```python
from build123d import *

# Parameters (mm, degrees)
SKETCH_1_R          = 5
EXTRUDE_1_DEPTH     = 5
CUT_EXTRUDE_1_DEPTH = 102.523396318


with BuildPart() as part:
    # 草图1 → 凸台-拉伸1 (new body)
    with BuildSketch(Plane.XY):
        with BuildLine():
            Line((0, 9), (92, 9))
            ThreePointArc((92, 9), (101, 0), (92, -9))
            Line((92, -9), (0, -9))
            ThreePointArc((0, -9), (-9, 0), (0, 9))
        make_face()
        Circle(SKETCH_1_R, mode=Mode.SUBTRACT)
        with Locations((92, 0)):
            Circle(SKETCH_1_R, mode=Mode.SUBTRACT)
    extrude(amount=EXTRUDE_1_DEPTH)

    # 草图2 → 切除-拉伸1 (cut, through all)
    with BuildSketch(Plane.XY.offset(5)):
        with BuildLine():
            Line((9.539392014, 4), (82.460607986, 4))
            ThreePointArc((82.460607986, 4), (83.266833761, 3.591607978), (83.414547187, 2.7))
            ThreePointArc((83.414547187, 2.7), (83, 0), (83.414547187, -2.7))
            ThreePointArc((83.414547187, -2.7), (83.266833761, -3.591607978), (82.460607986, -4))
            Line((82.460607986, -4), (9.539392014, -4))
            ThreePointArc((9.539392014, -4), (8.733166239, -3.591607978), (8.585452813, -2.7))
            ThreePointArc((8.585452813, -2.7), (9, 0), (8.585452813, 2.7))
            ThreePointArc((8.585452813, 2.7), (8.733166239, 3.591607978), (9.539392014, 4))
        make_face()
    extrude(amount=-CUT_EXTRUDE_1_DEPTH, mode=Mode.SUBTRACT)


solid = part.part
```
Work out the finished part from the listing and answer in its coordinate system (mm). A direction names the side the tool comes from. Give positions to 0.01 mm unless a question says otherwise; leave off trailing zeros. Loops run counter-clockwise (first coordinate to the right, second up) from the corner with the lowest first, then second, coordinate; pieces in that order, holes last. Notation, with made-up numbers: (-30, 10) - (22, 10) arc R31 ccw to (22, 46) - close; hole circle Ø6 at (49, -35.75). An arc over 180 degrees is marked (long way). Use CSV: the item, a comma, the result in double quotes. Start each with the question number.
(1) Find section A-A, the plane x = 73.5. Determine the outline of the cut face in (y, z).
(2) A tool of negligible diameter and unlimited length cuts with its end or side. For faces 1 (the face through (45, 4, 3)), 2 (the face through (47, 6, 5)), from which of +Z, -Z, +X, -X, +Y, -Y can it reach the whole face along a straight path? Write none if from no direction.
(3) Find section B-B, the plane y = 0. Determine the outline of the cut face in (x, z), plus the area to 3 significant figures.
(4) Find section C-C, the plane z = 3.4. Determine the outline of the cut face in (x, y), plus the area to 3 significant figures.
(5) Determine the mould class of faces 3 (the face through (9, 0, 3)), 4 (the face through (-1.08, -4.88, 2.46)), 5 (the face through (101, 0, 2)), 6 (the face through (47, -9, 2)) for opening direction Y: released by +Y, released by -Y, zero draft, split by the parting line, or undercut.
(6) Find section D-D, the plane x = 90. Determine the outline of the cut face in (y, z).
(7) Find the intervals of material crossed by L1, parallel to Y at x = 41.5, z = 3; L2, parallel to Y at x = 92, z = 2.5; L3, parallel to X at y = -3.5, z = 4.6, in increasing order.
Results found:
1,outline,"(-9, 0) - (-4, 0) - (-4, 5) - (-9, 5) - close; (4, 0) - (9, 0) - (9, 5) - (4, 5) - close"
2,face 1,"+Z, -Z"
2,face 2,"+Z, +X, -X, +Y, -Y"
3,outline,"(-9, 0) - (-5, 0) - (-5, 5) - (-9, 5) - close; (5, 0) - (9, 0) - (9, 5) - (5, 5) - close; (83, 0) - (87, 0) - (87, 5) - (83, 5) - close; (97, 0) - (101, 0) - (101, 5) - (97, 5) - close"
3,area,"80.0 mm^2"
4,outline,"(0, -9) - (92, -9) arc R9 ccw to (92, 9) - (0, 9) arc R9 ccw to start; hole circle Ø10 at (0, 0); hole (8.59, -2.7) arc R1 ccw to (9.54, -4) - (82.46, -4) arc R1 ccw to (83.41, -2.7) arc R9 cw to (83.41, 2.7) arc R1 ccw to (82.46, 4) - (9.54, 4) arc R1 ccw to (8.59, 2.7) arc R9 cw to start; hole circle Ø10 at (92, 0)"
4,area,"1,160 mm^2"
5,face 3,"undercut"
5,face 4,"undercut"
5,face 5,"split by the parting line"
5,face 6,"released by -Y"
6,outline,"(-9, 0) - (-4.58, 0) - (-4.58, 5) - (-9, 5) - close; (4.58, 0) - (9, 0) - (9, 5) - (4.58, 5) - close"
7,L1,"-9 to -4, 4 to 9"
7,L2,"-9 to -5, 5 to 9"
7,L3,"-8.29 to -3.57, 3.57 to 8.67, 83.33 to 88.43, 95.57 to 100.29"
